Here's how the part is built. I have some questions about the finished solid (model axes, mm). A direction names the side the tool comes from. Round coordinates to 2 decimals unless told otherwise and drop trailing zeros. Write each loop counter-clockwise with the first axis right and the second up, starting at its lowest first coordinate (ties: lowest second). Pieces come first, ordered by that corner, then holes. Notation, with made-up numbers: (-14.75, -10.5) -> (28.25, -10.5) arc R10 cw to (28.25, 8.5) -> close; hole circle Ø2 at (83.25, 66.5). An arc over 180 degrees is marked (long way). Answer as CSV lines item,"result".
Autodesk Fusion 360 part; units mm, degrees
sketch "Sketch1" plane through (0, 0, 0) normal (0, 0, 1) x (1, 0, 0) in component "Jewelry Sawing Block"
  line L0 (-30, 97.5) -> (30, 97.5)
  line L1 (30, 97.5) -> (30, -97.5)
  line L2 (30, -97.5) -> (-30, -97.5)
  line L3 (-30, -97.5) -> (-30, 97.5)
  line L4 (-30, 97.5) -> (30, -97.5) construction
  line L5 (30, 97.5) -> (-30, -97.5) construction
  circle A0 centre (0, 40) radius 8
  line L6 (0, 0) -> (0, 40) construction
  line L7 (-8, 97.5) -> (-8, 40)
  line L8 (8, 97.5) -> (8, 40)
  circle A1 centre (0, -35) radius 8
  line L9 (0, 0) -> (0, -35) construction
  line L10 (-22.5, -97.5) -> (-5.5, -40.8095)
  line L11 (22.5, -97.5) -> (5.5, -40.8095)
  dimension "d1" = 195
  dimension "d2" = 60
  dimension "d3" = 16
  dimension "d4" = 40
  dimension "d5" = 16
  dimension "d6" = 35
  dimension "d7" = 7.5
  dimension "d8" = 11
extrude "Extrude1" add sketch "Sketch1" along normal blind 8 contours L0 L1 L2 L3 A0 L7 L8 A1 L10 L11 | L0 A0 L7 L8 in component "Jewelry Sawing Block"
extrude "Extrude2" cut sketch "Sketch1" along normal blind 3 contours L0 A0 L7 L8 in component "Jewelry Sawing Block"
fillet "Fillet1" radius 3 4 edges at (-30, -97.5, 4) (30, -97.5, 4) (30, 97.5, 4) (-30, 97.5, 4) in component "Jewelry Sawing Block"
chamfer "Chamfer1" distance 1 angle 45 19 edges at (30, 0, 0) (29.1213, -96.6213, 0) (24.75, -97.5, 0) (17.5, 97.5, 0) (29.1213, 96.6213, 0) (-30, 0, 0) (-29.1213, 96.6213, 0) (-17.5, 97.5, 0) (-24.75, -97.5, 0) (-29.1213, -96.6213, 0) (30, 0, 8) (29.1213, 96.6213, 8) (0, 97.5, 8) (-29.1213, 96.6213, 8) (-30, 0, 8) (-29.1213, -96.6213, 8) (-24.75, -97.5, 8) (24.75, -97.5, 8) (29.1213, -96.6213, 8) in component "Jewelry Sawing Block"
component "Jewelry Sawing Block" placed x (1, 0, 0) y (0, 1, 0) z (0, 0, 1) at (0, 0, 0)
1. Suppose I cut it at D-D on x = 19. Please give me the cut outline in (y, z).
Numbers:
outline,"(-85.83, 0) -> (96.5, 0) -> (97.5, 1) -> (97.5, 7) -> (96.5, 8) -> (-85.83, 8) -> close"
2. For pin 1 Ø13 at (x, y) = (-1, 72.5) entering from -Z; pin 2 Ø14.5 at (x, y) = (0, -35) entering from -Z, each with a flat end and sliding along its axis, tell me the tip position at first contact or that it passes through.
Numbers:
pin 1,"stops at z = 3"
pin 2,"passes through"
3. Suppose I cut it at B-B on x = 0. Please give me the cut outline in (y, z), and give its area (3 significant figures).
Numbers:
outline,"(-27, 0) -> (32, 0) -> (32, 8) -> (-27, 8) -> close; (48, 3) -> (97.5, 3) -> (97.5, 7) -> (96.5, 8) -> (48, 8) -> close"
area,"719 mm^2"
4. Suppose I cut it at C-C on y = 60. Please give me the cut outline in (x, z).
Numbers:
outline,"(-30, 1) -> (-29, 0) -> (-8, 0) -> (-8, 3) -> (8, 3) -> (8, 0) -> (29, 0) -> (30, 1) -> (30, 7) -> (29, 8) -> (-29, 8) -> (-30, 7) -> close"
5. Suppose I cut it at A-A on y = -35. Please give me the cut outline in (x, z), and give its area (3 significant figures).
Numbers:
outline,"(-30, 1) -> (-29, 0) -> (-8, 0) -> (-8, 8) -> (-29, 8) -> (-30, 7) -> close; (8, 0) -> (29, 0) -> (30, 1) -> (30, 7) -> (29, 8) -> (8, 8) -> close"
area,"350 mm^2"
6. On a 3-axis mill with a long thin cutter (end or side, diameter ignored), from which of +Z, -Z, +X, -X, +Y, -Y can I reach the whole of each face in a straight line? I mean faces 5 (the face through (-25, -97.5, 4)), 6 (the face through (0, 69, 3)), 7 (the face through (14.12, -69.55, 3.94)). Say none if no direction works.
Numbers:
face 5,"+Z, -Z, +X, -X, -Y"
face 6,"-Z, +Y"
face 7,"+Z, -Z, -Y"
7. If we mould it in two halves opening along X, with no side actions, what happens to faces 1 (the face through (-30, -1, 4)), 2 (the face through (30, 1, 4)), 3 (the face through (-1.041, 32.068, 4.833)), 4 (the face through (0, 1, 8))? For each: released by +X, released by -X, zero draft, split by the parting line, or undercut.
Numbers:
face 1,"released by -X"
face 2,"released by +X"
face 3,"undercut"
face 4,"zero draft"
8. If I drill on line 1 (X direction, y = 40, z = 2.25); line 2 (Y direction, x = 0, z = 5); line 3 (X direction, y = -65.5, z = 3.5), over which ranges is the centre line in solid material (lowest first)?
Numbers:
line 1,"x = -30 to -8, 8 to 30"
line 2,"y = -27 to 32, 48 to 97.5"
line 3,"x = -30 to -12.9, 12.9 to 30"
